Autodesk Inventor part; units mm, degrees
ref_plane "YZ Plane" through (0, 0, 0) normal (1, 0, 0) x (0, 1, 0)
ref_plane "XZ Plane" through (0, 0, 0) normal (0, 1, 0) x (-1, 0, 0)
ref_plane "XY Plane" through (0, 0, 0) normal (0, 0, 1) x (1, 0, 0)
sketch "Sketch1" plane through (0, 0, 0) normal (0, 0, 1) x (1, 0, 0)
  line L0 (0, 0) -> (79.9084, 0)
  line L1 (79.9084, 0) -> (79.9084, 219.6084)
  line L2 (79.9084, 219.6084) -> (0, 219.6084)
  line L3 (0, 219.6084) -> (0, 0)
  dimension "d0" = 79.9084
  dimension "d1" = 219.6084
extrude "Extrusion1" add sketch "Sketch1" along normal blind 76.2
sketch "Sketch2" plane through (0, 0, 0) normal (0, -1, 0) x (1, 0, 0)
  line L0 (79.9084, 0) -> (79.9084, 76.2)
  line L1 (0, 0) -> (79.9084, 0)
  line L2 (0, 76.2) -> (79.9084, 76.2)
  line L3 (78.0542, 1.8542) -> (1.8542, 1.8542)
  line L4 (1.8542, 1.8542) -> (1.8542, 76.2)
  line L5 (1.8542, 76.2) -> (78.0542, 76.2)
  line L6 (78.0542, 76.2) -> (78.0542, 1.8542)
  dimension "d4" = 1.8542
  dimension "d5" = 1.8542
  dimension "d6" = 76.2
extrude "Extrusion2" cut sketch "Sketch2" against normal blind 228.6
sketch "Sketch3" plane through (0, 0, 76.2) normal (0, 0, 1) x (1, 0, 0)
  line L0 (1.8542, 0) -> (1.8542, 219.6084)
  line L1 (0, 219.6084) -> (1.8542, 219.6084)
  line L2 (1.8542, 219.6084) -> (1.8542, 143.4084)
  line L3 (1.8542, 143.4084) -> (0, 143.4084)
  line L4 (0, 143.4084) -> (0, 219.6084)
  point P0 (0, 0)
  dimension "d9" = 76.2
extrude "Extrusion3" cut sketch "Sketch3" against normal blind 74.3458
sketch "Sketch9" plane through (0, 0, 76.2) normal (0, 0, 1) x (1, 0, 0)
  line L0 (78.0542, 219.6084) -> (78.0542, 0)
  line L1 (0, 143.4084) -> (0, 219.6084)
  arc A0 (78.0542, 139.6114) -> (0, 217.6656) centre (0.5141, 140.1255) ccw
  line L2 (0, 217.6656) -> (78.0542, 139.6114) construction
  line L3 (0, 217.6656) -> (110.3853, 217.6656) construction
  line L4 (78.0542, 139.6114) -> (76.2, 139.6114)
  line L5 (0, 217.6656) -> (0, 215.8114)
  arc A1 (76.2, 139.6114) -> (0, 215.8114) centre (0.257, 139.8685) ccw
  point P0 (0, 0)
  dimension "d22" = 45
  dimension "d23" = 1.8542
  dimension "d24" = 1.8542
extrude "Extrusion7" add sketch "Sketch9" against normal blind 12.7
sketch "Sketch10" plane through (0, 0, 0) normal (-1, 0, 0) x (0, 0, 1)
  line L0 (0, 0) -> (76.2, 0)
  line L1 (76.2, 143.4084) -> (76.2, 0)
  point P0 (64.9986, 18.5674)
  point P1 (68.8594, 29.21)
  dimension "d27" = 18.5674
  dimension "d28" = 11.2014
  dimension "d29" = 7.3406
  dimension "d30" = 29.21
hole "Hole1" at (0, 29.21, 68.8594) at (0, 18.5674, 64.9986) direction (1, 0, 0) diameter 3.7084 depth 1.8542
sketch "Sketch11" plane through (79.9084, 0, 0) normal (1, 0, 0) x (0, 0, -1)
  line L0 (0, 0) -> (-76.2, 0)
  line L1 (-76.2, 0) -> (-76.2, 219.6084)
  point P0 (-70.7898, 40.1574)
  point P1 (-64.0842, 21.7678)
  dimension "d38" = 40.1574
  dimension "d39" = 5.4102
  dimension "d40" = 12.1158
  dimension "d41" = 21.7678
hole "Hole2" at (79.9084, 40.1574, 70.7898) at (79.9084, 21.7678, 64.0842) direction (-1, 0, 0) diameter 3.7084 depth 1.8542
properties part number "Sorter" material "Aluminum 6061"
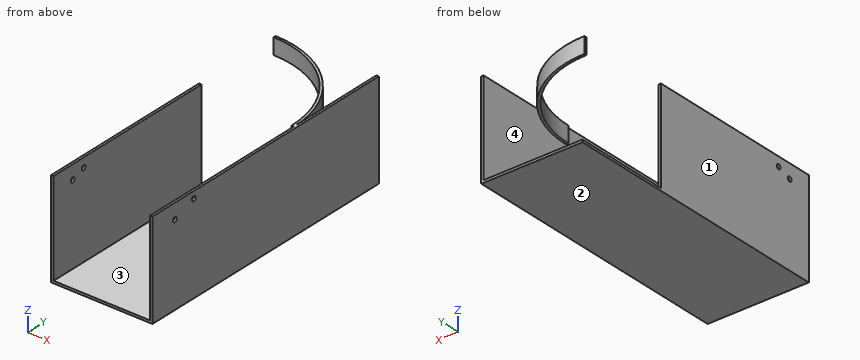
Can you work these out from the model? Positions are in its coordinate system, mm. Face numbers are marked on the shaded views. Coordinates: 2 decimals unless noted, no trailing zeros. Order: outer loops, then holes, each group sorted by start corner. A loop starts at its lowest first (then second) coordinate and runs counter-clockwise, first axis right, second up. Notation, with made-up numbers: (-13, -15.75) - (-9, -15.75) arc R22 ccw to (-9, 16.25) - close; hole circle Ø10 at (-16.5, 38.5). An arc over 180 degrees is marked (long way). Answer as a JSON object with one key per item and string values. Group by question number.
Q1. Will these pins go through, and if not, where does the flat tip stop? P1, Ø0.9, axis at x = 0.5, z = 45, coming from the +Y side; P2, Ø12, axis at x = 50.5, y = 23.5, coming from the +Z side; P3, Ø5, axis at y = 185.5, z = 66.5, coming from the -X side.
Q2. I need wall thicknesses on line 1 (X direction, y = 37.5, z = 64); line 2 (Z direction, x = 1.35, y = 29.21); line 3 (Z direction, x = 41, y = 143). Which ranges of each line are inside material? Lowest first, please. Write a range as from..to.
Q3. Imagine slicing it at B-B (y = 181.5). Please give me the cut outline in (x, z), and give its area (3 significant figures).
Q4. Imagine slicing it at C-C (z = 55). Please give me the cut outline in (x, y).
Q5. We'd pull the mould along X, two halves only. Please class the marked faces 1, 2, 3 and 4: +X half, -X half, draft (parallel to the pull), parting line (faces both ways), or undercut.
Q6. Imagine slicing it at D-D (y = 154.5). Please give me the cut outline in (x, z), and give its area (3 significant figures).
Q7. Imagine slicing it at A-A (x = 40). Please give me the cut outline in (y, z).
Determined:
{
 "1": {"P1": "stops at y = 143.41", "P2": "stops at z = 1.85", "P3": "stops at x = 59"},
 "2": {"line 1": "x = 0..1.85, 78.05..79.91", "line 2": "z = 0..67.01, 70.71..76.2", "line 3": "z = 0..1.85"},
 "3": {"outline": "(0, 0) - (79.91, 0) - (79.91, 76.2) - (78.05, 76.2) - (78.05, 1.85) - (0, 1.85) - close; (63.77, 63.5) - (66.1, 63.5) - (66.1, 76.2) - (63.77, 76.2) - close", "area": "316 mm2"},
 "4": {"outline": "(0, 0) - (1.85, 0) - (1.85, 143.41) - (0, 143.41) - close; (78.05, 0) - (79.91, 0) - (79.91, 219.61) - (78.05, 219.61) - close"},
 "5": {"face 1": "-X half", "face 2": "draft", "face 3": "undercut", "face 4": "undercut"},
 "6": {"outline": "(0, 0) - (79.91, 0) - (79.91, 76.2) - (78.05, 76.2) - (78.05, 1.85) - (0, 1.85) - close; (74.78, 63.5) - (76.71, 63.5) - (76.71, 76.2) - (74.78, 76.2) - close", "area": "311 mm2"},
 "7": {"outline": "(0, 0) - (219.61, 0) - (219.61, 1.85) - (0, 1.85) - close; (204.58, 63.5) - (206.86, 63.5) - (206.86, 76.2) - (204.58, 76.2) - close"}
}
